Check sheet for the modelled part. Datum: model origin and axes. Units: mm. Round coordinates to 2 decimals unless told otherwise and drop trailing zeros. Loops run counter-clockwise (first coordinate to the right, second up) from the corner with the lowest first, then second, coordinate; pieces in that order, holes last. Notation, with made-up numbers: (22, 20) - (70, 20) arc R24 cw to (70, 57) - close; hole circle Ø11 at (-17, 35). An arc over 180 degrees is marked (long way). Put each result on its own line as item: value.
```python
from build123d import *

# Parameters (mm, degrees)
F0_R     = 3.175
F1_DEPTH = 1.524


with BuildPart() as f1:
    # F0 (on Front) → F1 (new body, symmetric)
    with BuildSketch(Plane.XZ):
        with BuildLine():
            ThreePointArc((-2.38125, 41.577458), (5.832848, 43.269826), (9.525, 50.8))
            ThreePointArc((9.525, 50.8), (0, 60.325), (-9.525, 50.8))
            ThreePointArc((-9.525, 50.8), (-7.530174, 44.967152), (-2.38125, 41.577458))
        make_face()
        with Locations((0, 50.8)):
            Circle(F0_R, mode=Mode.SUBTRACT)
        with BuildLine():
            Line((15.747457, 2.008289), (9.525, 50.8))
            ThreePointArc((9.525, 50.8), (5.832848, 43.269826), (-2.38125, 41.577458))
            ThreePointArc((-2.38125, 41.577458), (-7.530174, 44.967152), (-9.525, 50.8))
            Line((-9.525, 50.8), (-15.747457, 2.008289))
            ThreePointArc((-15.747457, 2.008289), (0, 15.875), (15.747457, 2.008289))
        make_face()
        with BuildLine():
            ThreePointArc((0, 38.503278), (-5.685058, 36.558995), (-2.38125, 41.577458))
            ThreePointArc((-2.38125, 41.577458), (-0.664942, 40.44756), (0, 38.503278))
        make_face(mode=Mode.SUBTRACT)
        with BuildLine():
            ThreePointArc((15.875, 0), (15.843082, 1.006168), (15.747457, 2.008289))
            ThreePointArc((15.747457, 2.008289), (0, 15.875), (-15.747457, 2.008289))
            ThreePointArc((-15.747457, 2.008289), (-15.875, 0), (-15.747457, -2.008289))
            ThreePointArc((-15.747457, -2.008289), (0, -15.875), (15.747457, -2.008289))
            ThreePointArc((15.747457, -2.008289), (15.843082, -1.006168), (15.875, 0))
        make_face()
        Circle(F0_R, mode=Mode.SUBTRACT)
        with BuildLine():
            ThreePointArc((15.747457, -2.008289), (0, -15.875), (-15.747457, -2.008289))
            Line((-15.747457, -2.008289), (-9.525, -63.5))
            ThreePointArc((-9.525, -63.5), (0, -53.975), (9.525, -63.5))
            ThreePointArc((9.525, -63.5), (6.96982, -69.99209), (0.675187, -73.001039))
            Line((0.675187, -73.001039), (44.731685, -71.437583))
            ThreePointArc((44.731685, -71.437583), (36.50742, -63.5), (44.731685, -55.562417))
            Line((44.731685, -55.562417), (17.785491, -54.606163))
            ThreePointArc((17.785491, -54.606163), (12.008562, -51.808352), (10.18112, -45.655213))
            Line((10.18112, -45.655213), (15.747457, -2.008289))
        make_face()
        with BuildLine():
            ThreePointArc((9.525, -63.5), (0, -53.975), (-9.525, -63.5))
            ThreePointArc((-9.525, -63.5), (-6.735192, -70.235192), (0, -73.025))
            Line((0, -73.025), (0.675187, -73.001039))
            ThreePointArc((0.675187, -73.001039), (6.96982, -69.99209), (9.525, -63.5))
        make_face()
        with Locations((0, -63.5)):
            Circle(F0_R, mode=Mode.SUBTRACT)
        with BuildLine():
            Line((0.675187, -73.001039), (0, -73.025))
            ThreePointArc((0, -73.025), (0.337806, -73.019008), (0.675187, -73.001039))
        make_face()
        with BuildLine():
            ThreePointArc((52.39258, -63.5), (50.164975, -57.984238), (44.731685, -55.562417))
            ThreePointArc((44.731685, -55.562417), (36.50742, -63.5), (44.731685, -71.437583))
            ThreePointArc((44.731685, -71.437583), (50.164975, -69.015762), (52.39258, -63.5))
        make_face()
        with Locations((44.45, -63.5)):
            Circle(F0_R, mode=Mode.SUBTRACT)
    extrude(amount=F1_DEPTH, both=True)


solid = f1.part
```
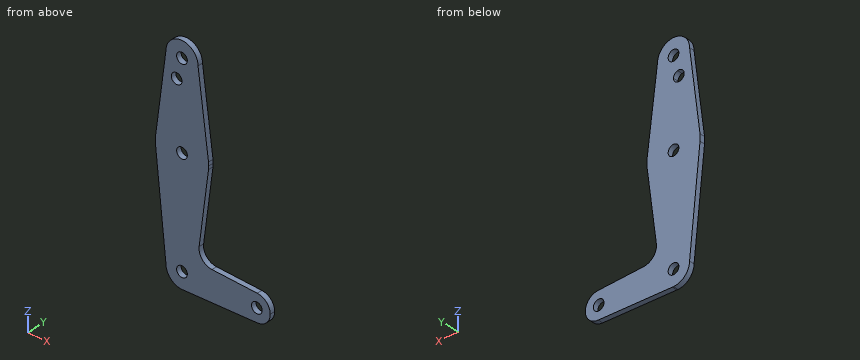
Item 1: Thickness scan on line 1 (Z direction, x = 44.5, y = -1); line 2 (Z direction, x = -5, y = 0.1); line 3 (Z direction, x = 2.5, y = 0.65). Record the ranges inside material, lowest first. Write a range as from..to.
Filled sheet:
line 1: -71.45..-66.67, -60.33..-55.55
line 2: -71.61..35.91, 41.1..58.91
line 3: -72.94..-65.46, -61.54..-1.96, 1.96..48.84, 52.76..59.99
Item 2: Section check A-A on y = -0.3. Count the separate pieces of the cut face and the enclosed holes in it, then the cut area to 3 significant figures.
Filled sheet:
separate pieces: 1
enclosed holes: 5
area: 3,730 mm²
Item 3: Go/stop test with flat-tipped pins: pin 1 (1 mm diameter, centred on y = -1, z = -17, fed in from +X); pin 2 (1 mm diameter, centred on x = 45, y = -1, fed in from -Z); pin 3 (1 mm diameter, centred on x = -5, y = 0, fed in from -Z) (3 decimals). Record where each tip stops, or that it passes through.
Filled sheet:
pin 1: x = 13.9
pin 2: z = -71.45
pin 3: z = -71.895
Item 4: Section check C-C on x = 28. Enter the section's corners in (y, z).
Filled sheet:
outline: (-1.52, -72.03) - (1.52, -72.03) - (1.52, -54.97) - (-1.52, -54.97) - close
Item 5: Section check B-B on z = 21.5. Enter the section's corners in (x, y), then the cut area to 3 significant figures.
Filled sheet:
outline: (-13.26, -1.52) - (13.26, -1.52) - (13.26, 1.52) - (-13.26, 1.52) - close
area: 80.8 mm²
